Here's how the part is built. I have some questions about the finished solid (model axes, mm). A direction names the side the tool comes from. Coordinates: 2 decimals unless noted, no trailing zeros. Write each loop counter-clockwise with the first axis right and the second up, starting at its lowest first coordinate (ties: lowest second). Pieces come first, ordered by that corner, then holes. Notation, with made-up numbers: (89.25, 54.25) -> (148.25, 54.25) arc R32 ccw to (148.25, 89.25) -> close; hole circle Ø5 at (10.5, 3.5). An arc over 180 degrees is marked (long way). Put each result on its own line as item: value. Start each with the question number.
Item 1: On a 3-axis mill with a long thin cutter (end or side, diameter ignored), from which of +Z, -Z, +X, -X, +Y, -Y can I reach the whole of each face in a straight line? I mean faces 5 (the face through (-0.71, 7.91, -2.24)), 6 (the face through (16.93, 0.02, 16.9)). Say none if no direction works.
Item 2: I want a section at A-A, the plane x = 15. List the corners of the cut face in (y, z) for me, then the cut area to 3 significant figures.
Item 3: If we mould it in two halves opening along Z, with no side actions, what happens to faces 1 (the face through (-15.43, 0.02, 13.64)), 2 (the face through (14.415, 0.021, -12.534)), 3 (the face through (0, 0, 17.5)), 4 (the face through (-16.93, -0.02, -16.9))? For each: released by +Z, released by -Z, zero draft, split by the parting line, or undercut.
Item 4: I want a section at B-B, the plane z = 0. List the corners of the cut face in (x, y) for me.
Item 5: I need wall thicknesses on line 1 (Y direction, x = 3, z = -4.5); line 2 (X direction, y = 0.5, z = 13.5); line 3 (Z direction, x = -2, y = 6.5). Which ranges of each line are inside material? Lowest first, please. Write a range as [from, to].
Item 6: For pin 1 (3.5 mm diameter, centred on x = -13.96, z = 13.96, fed in from -Y); pin 2 (3.5 mm diameter, centred on x = -13.96, z = -13.96, fed in from +Y); pin 3 (4 mm diameter, centred on x = -2.5, y = 7, fed in from -Z), each with a flat end and sliding along its axis, tell me the tip position at first contact or that it passes through.
Item 7: I want a section at D-D, the plane z = 15. List the corners of the cut face in (x, y) for me.
Item 8: I want a section at C-C, the plane y = 1. List the corners of the cut face in (x, z) for me.
from build123d import *

# Parameters (mm, degrees)
ESBO_O1_W                = 35
ESBO_O1_H                = 35
RESSALTO_EXTRUS_O1_DEPTH = 1.5
FILETE1_R                = 2
ESBO_O2_R                = 2.35
RESSALTO_EXTRUS_O2_DEPTH = 13
ESBO_O3_R                = 1.5
CORTE_EXTRUS_O1_DEPTH    = 10


with BuildPart() as part:
    # Esboço1 → Ressalto-extrusão1 (new, symmetric)
    with BuildSketch(Plane(origin=(0, 0, 0), x_dir=(1, 0, 0), z_dir=(0, 1, 0))):
        Rectangle(ESBO_O1_W, ESBO_O1_H)
    extrude(amount=RESSALTO_EXTRUS_O1_DEPTH, both=True)

    # Filete1
    filete1_edges = [part.edges().sort_by_distance(p)[0] for p in [
        (17.5, 0, 17.5),
        (-17.5, 0, 17.5),
        (-17.5, 0, -17.5),
        (17.5, 0, -17.5),
    ]]
    fillet(filete1_edges, radius=FILETE1_R)

    # Esboço2 → Ressalto-extrusão2 (add)
    with BuildSketch(Plane(origin=(0, 1.5, 0), x_dir=(1, 0, 0), z_dir=(0, 1, 0))):
        with Locations(Location((0, 0, 0), (0, 0, 90))):
            Circle(ESBO_O2_R)
    extrude(amount=RESSALTO_EXTRUS_O2_DEPTH)

    # Esboço3 → Corte-extrusão1 (cut)
    with BuildSketch(Plane(origin=(0, 1.5, 0), x_dir=(1, 0, 0), z_dir=(0, 1, 0))):
        with Locations(Location((13.964466094, 13.964466094, 0), (0, 0, 270))):
            Circle(ESBO_O3_R)
        with Locations(Location((13.964466094, -13.964466094, 0), (0, 0, 270))):
            Circle(ESBO_O3_R)
        with Locations(Location((-13.964466094, -13.964466094, 0), (0, 0, 270))):
            Circle(ESBO_O3_R)
        with Locations(Location((-13.964466094, 13.964466094, 0), (0, 0, 270))):
            Circle(ESBO_O3_R)
    extrude(amount=-CORTE_EXTRUS_O1_DEPTH, mode=Mode.SUBTRACT)


solid = part.part
Calculated:
1. face 5: +Y
1. face 6: +Z, +X, +Y, -Y
2. outline: (-1.5, -17.5) -> (1.5, -17.5) -> (1.5, -15.05) -> (-1.5, -15.05) -> close; (-1.5, -12.88) -> (1.5, -12.88) -> (1.5, 12.88) -> (-1.5, 12.88) -> close; (-1.5, 15.05) -> (1.5, 15.05) -> (1.5, 17.5) -> (-1.5, 17.5) -> close
2. area: 92.0 mm2
3. face 1: undercut
3. face 2: undercut
3. face 3: released by +Z
3. face 4: released by -Z
4. outline: (-17.5, -1.5) -> (17.5, -1.5) -> (17.5, 1.5) -> (2.35, 1.5) -> (2.35, 14.5) -> (-2.35, 14.5) -> (-2.35, 1.5) -> (-17.5, 1.5) -> close
5. line 1: y = [-1.5, 1.5]
5. line 2: x = [-17.5, -15.39], [-12.54, 12.54], [15.39, 17.5]
5. line 3: z = [-1.23, 1.23]
6. pin 1: stops at y = -1.5
6. pin 2: stops at y = 1.5
6. pin 3: stops at z = -2.3
7. outline: (-17.5, -1.5) -> (-15.05, -1.5) -> (-15.05, 1.5) -> (-17.5, 1.5) -> close; (-12.88, -1.5) -> (12.88, -1.5) -> (12.88, 1.5) -> (-12.88, 1.5) -> close; (15.05, -1.5) -> (17.5, -1.5) -> (17.5, 1.5) -> (15.05, 1.5) -> close
8. outline: (-17.5, -15.5) arc R2 ccw to (-15.5, -17.5) -> (15.5, -17.5) arc R2 ccw to (17.5, -15.5) -> (17.5, 15.5) arc R2 ccw to (15.5, 17.5) -> (-15.5, 17.5) arc R2 ccw to (-17.5, 15.5) -> close; hole circle Ø3 at (-13.96, -13.96); hole circle Ø3 at (-13.96, 13.96); hole circle Ø3 at (13.96, -13.96); hole circle Ø3 at (13.96, 13.96)
